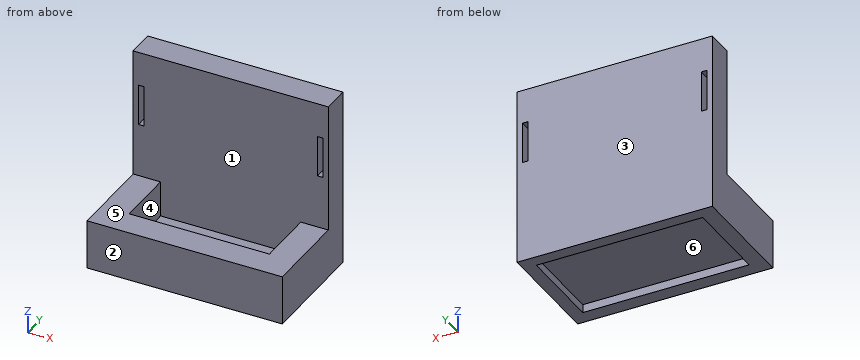
from build123d import *

# Parameters (mm, degrees)
F1_DEPTH = 18
F0_W     = 51
F0_H     = 21.5
F2_DEPTH = 5
F4_DEPTH = 47
F5_W     = 2
F5_H     = 12.5
F5_H_2   = 2.5
F6_DEPTH = 10
F7_W     = 60.499498
F7_H     = 31.819807
F8_DEPTH = 3


with BuildPart() as f1:
    # F0 (on Top) → F1 (new body)
    with BuildSketch(Plane.XY):
        Polygon((-37.291151, 13.41747), (-27.291151, 13.41747), (23.708849, 13.41747), (33.708849, 13.41747), (33.708849, 23.41747), (23.708849, 23.41747), (-27.291151, 23.41747), (-37.291151, 23.41747), align=None)
        Polygon((-27.291151, -8.08253), (-27.291151, 13.41747), (-37.291151, 13.41747), (-37.291151, -8.08253), (-37.291151, -18.08253), (-27.291151, -18.08253), (23.708849, -18.08253), (33.708849, -18.08253), (33.708849, -8.08253), (33.708849, 13.41747), (23.708849, 13.41747), (23.708849, -8.08253), align=None)
    extrude(amount=F1_DEPTH)

    # F0 (on Top) → F2 (join)
    with BuildSketch(Plane.XY):
        with Locations((-1.791151, 2.66747)):
            Rectangle(F0_W, F0_H)
    extrude(amount=F2_DEPTH)

    # F3 (on face) → F4 (join)
    with BuildSketch(Plane.XY.offset(18)):
        Polygon((33.708849, 23.41747), (-37.291151, 23.41747), (-37.291151, 13.41747), (-27.291151, 13.41747), (23.708849, 13.41747), (33.708849, 13.41747), align=None)
    extrude(amount=F4_DEPTH)

    # F5 (on face) → F6 (cut)
    with BuildSketch(Plane.XZ.offset(-13.41747)):
        Polygon((-33.291151, 37.5), (-33.291151, 50), (-33.291151, 52.5), (-35.291151, 52.5), (-35.291151, 37.5), align=None)
        with Locations((30.708849, 43.75)):
            Rectangle(F5_W, F5_H)
        with Locations((30.708849, 51.25)):
            Rectangle(F5_W, F5_H_2)
    extrude(amount=-F6_DEPTH, mode=Mode.SUBTRACT)

    # F7 (on face) → F8 (cut)
    with BuildSketch(Plane(origin=(0, 0, 0), x_dir=(1, 0, 0), z_dir=(0, 0, -1))):
        with Locations((-1.184429, -3.051597)):
            Rectangle(F7_W, F7_H)
    extrude(amount=-F8_DEPTH, mode=Mode.SUBTRACT)


solid = f1.part
Verification items for the finished model (mm, model axes). Face numbers are marked on the shaded views. A direction names the side the tool comes from. Give positions to 0.01 mm unless a question says otherwise; leave off trailing zeros. Loops run counter-clockwise (first coordinate to the right, second up) from the corner with the lowest first, then second, coordinate; pieces in that order, holes last. Notation, with made-up numbers: (69.5, -2) - (92.5, -2) arc R19 cw to (92.5, 35) - close; hole circle Ø4 at (9, 40.5). An arc over 180 degrees is marked (long way). Write item = value, one per line. Start each with the question number.
Q1. Tool access check on the marked faces 4, 5 and 6. Record the directions out of +Z, -Z, +X, -X, +Y, -Y that give a thin tool (end or side, any length) a straight path to the whole face; none if there is none.
Q2. Thickness scan on line 1 (X direction, y = 19, z = 38.5); line 2 (Y direction, x = 4, z = 14.5); line 3 (X direction, y = 7, z = 8). Record the ranges inside material, lowest first.
Q3. Cross-section at C-C, the plane z = 9.5. Enter the section's corners in (x, y).
Q4. Cross-section at D-D, the plane x = -21. Enter the section's corners in (y, z).
Q5. Depth check by flat-ended pin: P1, Ø1.6, axis at x = -34.5, y = 16.5, coming from the -Z side; P2, Ø1.5, axis at x = -20.5, y = -3, coming from the +Z side; P3, Ø6, axis at x = -20.5, z = 30.5, coming from the -Y side. Enter the tip coordinate at first touch or a pass-through.
Q6. Cross-section at B-B, the plane y = 18. Enter the section's corners in (x, z), and give its area (3 significant figures).
Q7. Cross-section at A-A, the plane z = 40. Enter the section's corners in (x, y).
Q8. Mould release check, pull along Y, two halves, no side actions. Record for the marked faces 1, 2 and 3: released by +Y, released by -Y, zero draft, split by the parting line, or undercut.
Answer key:
q1.face_4 = +Z
q1.face_5 = +Z, +X, -X, -Y
q1.face_6 = -Z
q2.line_1 = -37.29 to -35.29, -33.29 to 29.71, 31.71 to 33.71
q2.line_2 = -18.08 to -8.08, 13.42 to 23.42
q2.line_3 = -37.29 to -27.29, 23.71 to 33.71
q3.outline = (-37.29, -18.08) - (33.71, -18.08) - (33.71, 23.42) - (-37.29, 23.42) - close; hole (-27.29, -8.08) - (23.71, -8.08) - (23.71, 13.42) - (-27.29, 13.42) - close
q4.outline = (-18.08, 0) - (-12.86, 0) - (-12.86, 3) - (18.96, 3) - (18.96, 0) - (23.42, 0) - (23.42, 65) - (13.42, 65) - (13.42, 5) - (-8.08, 5) - (-8.08, 18) - (-18.08, 18) - close
q5.P1 = 0
q5.P2 = 5
q5.P3 = 13.42
q6.outline = (-37.29, 0) - (-31.43, 0) - (-31.43, 3) - (29.07, 3) - (29.07, 0) - (33.71, 0) - (33.71, 65) - (-37.29, 65) - close; hole (-35.29, 37.5) - (-33.29, 37.5) - (-33.29, 52.5) - (-35.29, 52.5) - close; hole (29.71, 37.5) - (31.71, 37.5) - (31.71, 52.5) - (29.71, 52.5) - close
q6.area = 4,370 mm^2
q7.outline = (-37.29, 13.42) - (-35.29, 13.42) - (-35.29, 23.42) - (-37.29, 23.42) - close; (-33.29, 13.42) - (29.71, 13.42) - (29.71, 23.42) - (-33.29, 23.42) - close; (31.71, 13.42) - (33.71, 13.42) - (33.71, 23.42) - (31.71, 23.42) - close
q8.face_1 = undercut
q8.face_2 = released by -Y
q8.face_3 = released by +Y
